Check sheet for the modelled part. Datum: model origin and axes. Units: mm. A direction names the side the tool comes from. Coordinates: 2 decimals unless noted, no trailing zeros. Write each loop counter-clockwise with the first axis right and the second up, starting at its lowest first coordinate (ties: lowest second). Pieces come first, ordered by that corner, then holes. Notation, with made-up numbers: M 11,-22.5 L 44,-22.5 A18 ccw 44,-3.5 Z; hole C -26.5,48 d8. An arc over 180 degrees is marked long. Answer as CSV lines item,"result". Start each with the question number.
Q1. Thickness scan on line 1 along X through (y, z) = (2.25, 1.25) (3 decimals); line 2 along Z through (x, y) = (-2.5, 0.5). Record the ranges inside material, lowest first. Write a range as from..to.
Q2. Mould release check, pull along Y, two halves, no side actions. Record for faces 5 (the flat face through (0, 10.16, 3)), 6 (the flat face through (0, -10.16, 3)), 7 (the flat face through (0, 0, 0)): pulls with the +Y half, pulls with the -Y half, needs draft (parallel to the pull), parting line crosses it, or undercut.
Q3. Sectioned sample at B-B, the plane z = 0.75. Record the cut outline in (x, y) (3 decimals).
Q4. Sectioned sample at A-A, the plane x = 6.75. Record the cut outline in (y, z) (3 decimals), then the cut area to 3 significant figures.
Q5. Access from +Z, -Z, +X, -X, +Y, -Y to the whole of each face (thin tool, end or side, straight path). Record for faces 1 (the flat face through (5, -0.635, 3)), 2 (the flat face through (5, 0.635, 3)), 3 (the flat face through (-0.635, 5, 3)), 4 (the flat face through (-5, -0.635, 3)).
Q6. Depth check by flat-ended pin: pin 1 Ø3 at (x, y) = (-3, 5) entering from +Z; pin 2 Ø2.5 at (x, z) = (5, 4.5) entering from +Y (3 decimals); pin 3 Ø2.5 at (y, z) = (3.5, 2.5) entering from +X (3 decimals); pin 4 Ø1.6 at (y, z) = (6.5, 3.5) entering from -X (3 decimals). Enter the tip coordinate at first touch or a pass-through.
from build123d import *

# Parameters (mm, degrees)
F0_W     = 9.525
F0_H     = 1.27
F0_W_2   = 1.27
F0_H_2   = 9.525
F1_DEPTH = 6.35
F2_R     = 0.508


with BuildPart() as f1:
    # F0 (on Top) → F1 (new body)
    with BuildSketch(Plane.XY):
        with Locations((-5.3975, 0)):
            Rectangle(F0_W, F0_H)
        with Locations((0, 5.3975)):
            Rectangle(F0_W_2, F0_H_2)
        with Locations((5.3975, 0)):
            Rectangle(F0_W, F0_H)
        with Locations((0, -5.3975)):
            Rectangle(F0_W_2, F0_H_2)
        Rectangle(F0_W_2, F0_H)
    extrude(amount=F1_DEPTH)

    # F2
    f2_edges = [f1.edges().sort_by_distance(p)[0] for p in [
        (0.635, -5.3975, 6.35),
        (-0.635, -5.3975, 6.35),
        (-5.3975, -0.635, 6.35),
        (-5.3975, 0.635, 6.35),
        (-0.635, 5.3975, 6.35),
        (0.635, 5.3975, 6.35),
        (5.3975, 0.635, 6.35),
        (5.3975, -0.635, 6.35),
        (-5.3975, 0.635, 0),
        (-5.3975, -0.635, 0),
        (5.3975, -0.635, 0),
        (5.3975, 0.635, 0),
        (0.635, 5.3975, 0),
        (-0.635, 5.3975, 0),
        (-0.635, -5.3975, 0),
        (0.635, -5.3975, 0),
    ]]
    fillet(f2_edges, radius=F2_R)


solid = f1.part
Output:
1,line 1,"x = -0.635..0.635"
1,line 2,"z = 0.16..6.19"
2,face 5,"pulls with the +Y half"
2,face 6,"pulls with the -Y half"
2,face 7,"needs draft"
3,outline,"M -10.16,-0.635 L -0.635,-0.635 L -0.635,-10.16 L 0.635,-10.16 L 0.635,-0.635 L 10.16,-0.635 L 10.16,0.635 L 0.635,0.635 L 0.635,10.16 L -0.635,10.16 L -0.635,0.635 L -10.16,0.635 Z"
4,outline,"M -0.635,0.508 A0.508 ccw -0.127,0 L 0.127,0 A0.508 ccw 0.635,0.508 L 0.635,5.842 A0.508 ccw 0.127,6.35 L -0.127,6.35 A0.508 ccw -0.635,5.842 Z"
4,area,"7.84 mm^2"
5,face 1,"+Z, -Z, +X, -Y"
5,face 2,"+Z, -Z, +X, +Y"
5,face 3,"+Z, -Z, -X, +Y"
5,face 4,"+Z, -Z, -X, -Y"
6,pin 1,"passes through"
6,pin 2,"stops at y = 0.635"
6,pin 3,"stops at x = 0.635"
6,pin 4,"stops at x = -0.635"
